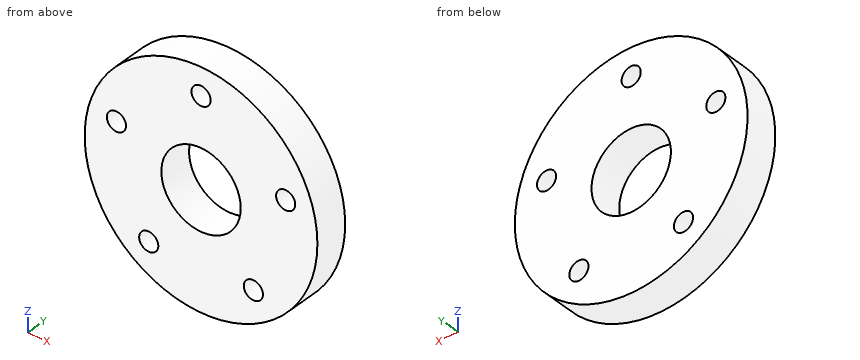
```python
from build123d import *

# Parameters (mm, degrees)
F0_R     = 85
F0_R_2   = 7
F0_R_3   = 29
F1_DEPTH = 25


# Not quite as in the source:
# - the program builds the solid bodies; features that only make, move or delete a surface that nothing else refers to are left out


with BuildPart() as f1:
    # F0 (on Front) → F1 (new body)
    with BuildSketch(Plane.XZ):
        Circle(F0_R)
        with Locations((-38.206041399, -52.5861046344)):
            Circle(F0_R_2, mode=Mode.SUBTRACT)
        with Locations((38.206041399, -52.5861046344)):
            Circle(F0_R_2, mode=Mode.SUBTRACT)
        with Locations((-61.8186735592, 20.0861046344)):
            Circle(F0_R_2, mode=Mode.SUBTRACT)
        Circle(F0_R_3, mode=Mode.SUBTRACT)
        with Locations((61.8186735592, 20.0861046344)):
            Circle(F0_R_2, mode=Mode.SUBTRACT)
        with Locations((0, 65)):
            Circle(F0_R_2, mode=Mode.SUBTRACT)
    extrude(amount=F1_DEPTH)


solid = f1.part
```
Work out the finished part from the listing and answer in its coordinate system (mm). Coordinates: 2 decimals unless noted, no trailing zeros. Write each loop counter-clockwise with the first axis right and the second up, starting at its lowest first coordinate (ties: lowest second). Pieces come first, ordered by that corner, then holes.
Q1. Find the intervals of material crossed by line 1 (Z direction, x = 0, y = -6.75); line 2 (Z direction, x = 4, y = -22); line 3 (Z direction, x = -11.5, y = -15), in increasing order.
Q2. A cutting plane is placed at D-D, the plane y = -13.75. Give the vertices of the cut face in (x, z), then the cut area to 3 significant figures.
Q3. A cutting plane is placed at B-B, the plane z = 0. Give the vertices of the cut face in (x, y).
Q4. Each of these flat-tipped pins is pushed along its axis until it touches: pin 1 Ø4 at (x, y) = (56, -16) entering from +Z; pin 2 Ø12 at (y, z) = (-10.5, 40.5) entering from -X; pin 3 Ø6 at (y, z) = (-9.5, -40) entering from -X. Where does it stop, or does it pass through?
Q5. A cutting plane is placed at C-C, the plane z = -48. Give the vertices of the cut face in (x, y).
Q6. A cutting plane is placed at A-A, the plane x = 0. Give the vertices of the cut face in (y, z), then the cut area to 3 significant figures.
Findings below:
1. line 1: z = -85 to -29, 29 to 58, 72 to 85
1. line 2: z = -84.91 to -28.72, 28.72 to 59.26, 70.74 to 84.91
1. line 3: z = -84.22 to -26.62, 26.62 to 84.22
2. outline: circle Ø170 at (0, 0); hole circle Ø14 at (-61.82, 20.09); hole circle Ø14 at (-38.21, -52.59); hole circle Ø58 at (0, 0); hole circle Ø14 at (0, 65); hole circle Ø14 at (38.21, -52.59); hole circle Ø14 at (61.82, 20.09)
2. area: 19,300 mm2
3. outline: (-85, -25) - (-29, -25) - (-29, 0) - (-85, 0) - close; (29, -25) - (85, -25) - (85, 0) - (29, 0) - close
4. pin 1: stops at z = 65.64
4. pin 2: stops at x = -77.68
4. pin 3: stops at x = -76.52
5. outline: (-70.15, -25) - (-43.49, -25) - (-43.49, 0) - (-70.15, 0) - close; (-32.92, -25) - (32.92, -25) - (32.92, 0) - (-32.92, 0) - close; (43.49, -25) - (70.15, -25) - (70.15, 0) - (43.49, 0) - close
6. outline: (-25, -85) - (0, -85) - (0, -29) - (-25, -29) - close; (-25, 29) - (0, 29) - (0, 58) - (-25, 58) - close; (-25, 72) - (0, 72) - (0, 85) - (-25, 85) - close
6. area: 2,450 mm2
